```python
from build123d import *

# Parameters (mm, degrees)
F0_W     = 50
F0_H     = 100
F1_DEPTH = 15
F2_R     = 10
F3_T     = 4.5


with BuildPart() as f1:
    # F0 (on Top) → F1 (new body)
    with BuildSketch(Plane.XY):
        with Locations((25, 50)):
            Rectangle(F0_W, F0_H)
    extrude(amount=F1_DEPTH)

    # F2
    f2_edges = [f1.edges().sort_by_distance(p)[0] for p in [
        (0, 0, 7.5),
        (50, 0, 7.5),
        (50, 100, 7.5),
        (0, 100, 7.5),
    ]]
    fillet(f2_edges, radius=F2_R)

    # F3
    f3_openings = [f1.faces().sort_by_distance(p)[0] for p in [
        (25, 50, 15),
    ]]
    offset(amount=F3_T, openings=f3_openings, kind=Kind.INTERSECTION)


solid = f1.part
```
Geometry: final body of the model. Coordinates: model frame, mm. A direction names the side the tool comes from. Round coordinates to 2 decimals unless told otherwise and drop trailing zeros. Loops run counter-clockwise (first coordinate to the right, second up) from the corner with the lowest first, then second, coordinate; pieces in that order, holes last.
Item 1: Section A-A, the plane z = 13. Output: boundary loops of the cut face in (x, y), plus the area to 3 significant figures.
Checked values:
outline: (-4.5, 10) arc R14.5 ccw to (10, -4.5) - (40, -4.5) arc R14.5 ccw to (54.5, 10) - (54.5, 90) arc R14.5 ccw to (40, 104.5) - (10, 104.5) arc R14.5 ccw to (-4.5, 90) - close; hole (0, 10) arc R10 ccw to (10, 0) - (40, 0) arc R10 ccw to (50, 10) - (50, 90) arc R10 ccw to (40, 100) - (10, 100) arc R10 ccw to (0, 90) - close
area: 1,340 mm2
Item 2: Section C-C, the plane x = 15. Output: boundary loops of the cut face in (y, z), plus the area to 4 significant figures.
Checked values:
outline: (-4.5, -4.5) - (104.5, -4.5) - (104.5, 15) - (100, 15) - (100, 0) - (0, 0) - (0, 15) - (-4.5, 15) - close
area: 625.5 mm2
Item 3: Section B-B, the plane z = -2. Output: boundary loops of the cut face in (x, y).
Checked values:
outline: (-4.5, 10) arc R14.5 ccw to (10, -4.5) - (40, -4.5) arc R14.5 ccw to (54.5, 10) - (54.5, 90) arc R14.5 ccw to (40, 104.5) - (10, 104.5) arc R14.5 ccw to (-4.5, 90) - close
Item 4: Mould query, pull axis Y, two halves, no side actions, for faces 1 (the flat face through (25, -4.5, 5)), 2 (the flat face through (-1, 46, 15)), 3 (the cylindrical face through (2.85, 96.99, 7.6)). Classes: released by +Y, released by -Y, zero draft, split by the parting line, or undercut.
Checked values:
face 1: released by -Y
face 2: zero draft
face 3: undercut
Item 5: Line query: L1, parallel to X at y = 46, z = 6.75; L2, parallel to Y at x = 15, z = 5.5; L3, parallel to Z at x = 25.5, y = 52. Output: solid intervals per line, ascending.
Checked values:
L1: x = -4.5 to 0, 50 to 54.5
L2: y = -4.5 to 0, 100 to 104.5
L3: z = -4.5 to 0
Item 6: Contact query for flat-ended pins moving along their axis: P1, Ø3, axis at x = 43.5, z = 7.5, coming from the -Y side; P2, Ø2, axis at x = 26.5, y = 37, coming from the +Z side. Output: stop coordinate, or through.
Checked values:
P1: stops at y = -4.36
P2: stops at z = 0
Item 7: Reachability of faces 4 (the flat face through (25, 100, 7)), 5 (the cylindrical face through (-0.365, -0.14, 5.386)) from +Z, -Z, +X, -X, +Y, -Y: full face, straight path, thin tool, end or side. Return the list, or none.
Checked values:
face 4: +Z
face 5: +Z, -Z, -X, -Y
